```python
from build123d import *

# Parameters (mm, degrees)
SKETCH_1_W          = 42.04
SKETCH_1_H          = 27.22
EXTRUDE_1_DEPTH     = 0.52
SKETCH_3_W          = 42.04
SKETCH_3_H          = 23.01
EXTRUDE_2_DEPTH     = 0.71
SKETCH_5_W          = 35.05
SKETCH_5_H          = 15.32
CUT_EXTRUDE_1_DEPTH = 0.01
EXTRUDE_START       = -6.26
EXTRUDE_1_2_DEPTH   = 12.52


# Read off the part's stored shape, not the designer's step: 拉伸-薄壁1
with BuildPart() as part:
    # 草图1 → Extrude 1 (new body)
    with BuildSketch(Plane.XY):
        Rectangle(SKETCH_1_W, SKETCH_1_H)
    extrude(amount=EXTRUDE_1_DEPTH)

    # 草图3 → 凸台-拉伸2 (add)
    with BuildSketch(Plane.XY):
        with Locations((0, 2.105)):
            Rectangle(SKETCH_3_W, SKETCH_3_H)
    extrude(amount=-EXTRUDE_2_DEPTH)

    # 草图5 → 切除-拉伸1 (cut)
    with BuildSketch(Plane.XY):
        with Locations((0, 2.105)):
            Rectangle(SKETCH_5_W, SKETCH_5_H)
    extrude(amount=-CUT_EXTRUDE_1_DEPTH, mode=Mode.SUBTRACT)

    # Extrude 1 2 outline → Extrude 1 2 (add)
    with BuildSketch(Plane(origin=(0, 0, 0), x_dir=(0, 0, -1), z_dir=(1, 0, 0)).offset(EXTRUDE_START)):
        with BuildLine():
            Line((0, -13.61), (-0.1, -13.61))
            add(Edge.make_bspline(
                [(-0.1, -13.61), (-0.1, -13.811999948), (-0.062447397, -13.983759134), (0.087597414, -14.266880112), (0.200229868, -14.375905512), (0.61293299, -14.604541747), (0.98162629, -14.634564325), (2.275338874, -14.53538179), (3.401387146, -14.206264697), (4.808904257, -13.842712132), (5.090182683, -13.77233657), (5.643385338, -13.645546605), (5.91499808, -13.589621122), (6.715455086, -13.444072044), (7.229865116, -13.376385405), (8.718879461, -13.254443705), (9.639245367, -13.281281386), (12.212088444, -13.631316764), (13.676832265, -14.22370802), (16.256955878, -15.84390487), (17.371964057, -16.872230984), (20.403860489, -20.184886502), (22.003130479, -22.695949544), (24.648389829, -25.189380489), (25.574110216, -25.809694734), (27.660843497, -26.317217871), (28.817134045, -26.200070844), (30.142790661, -25.575336117)],
                knots=[0, 0, 0, 0, 0.015625, 0.015625, 0.03125, 0.03125, 0.0625, 0.0625, 0.125, 0.125, 0.140625, 0.140625, 0.15625, 0.15625, 0.1875, 0.1875, 0.25, 0.25, 0.375, 0.375, 0.5, 0.5, 0.75, 0.75, 0.875, 0.875, 1, 1, 1, 1], degree=3))
            Line((30.142790661, -25.575336117), (30.100160891, -25.484877824))
            add(Edge.make_bspline(
                [(0, -13.61), (0, -15.345647415), (20.557920243, -6.954998075), (21.119775691, -29.717013379), (30.100160891, -25.484877824)],
                knots=[0, 0, 0, 0, 0.142988606, 1, 1, 1, 1], degree=3))
        make_face()
    extrude(amount=EXTRUDE_1_2_DEPTH)


solid = part.part
```
CAD build for the part. Positions are in the model's coordinates, mm. A direction names the side the tool comes from. Give positions to 0.01 mm unless a question says otherwise; leave off trailing zeros. Loops run counter-clockwise (first coordinate to the right, second up) from the corner with the lowest first, then second, coordinate; pieces in that order, holes last. Notation, with made-up numbers: (41.25, 64) -> (53.25, 64) arc R16 ccw to (53.25, 83) -> close; hole circle Ø2 at (70, -22.75). An arc over 180 degrees is marked (long way). Use a Markdown table: item, result.
1. Wall check: L1, parallel to Z at x = 13, y = -11; L2, parallel to Z at x = 13, y = 11.5; L3, parallel to Y at x = 3.5, z = -23. Give the ranges that are in metal, low to high. Write a range as [from, to].
Check result:
| item | result |
|---|---|
| L1 | z = [0, 0.52] |
| L2 | z = [-0.71, 0.52] |
| L3 | y = [-23.58, -23.43] |
2. Flat gauge pins, fed straight in: pin 1 (17 mm diameter, centred on x = 4.5, y = 2, fed in from -Z); pin 2 (14.5 mm diameter, centred on y = -21.5, z = -18.5, fed in from +X); pin 3 (3 mm diameter, centred on x = -6, z = -19.5, fed in from +Y). Where does each tip first touch, or does it go through?
Check result:
| item | result |
|---|---|
| pin 1 | stops at z = -0.71 |
| pin 2 | stops at x = 6.26 |
| pin 3 | stops at y = -17.42 |
3. Slice it at B-B (x = 7.5). List the corners of the cut face in (y, z) (3 decimals).
Check result:
| item | result |
|---|---|
| outline | (-13.61, 0) -> (-9.4, 0) -> (-9.4, -0.71) -> (13.61, -0.71) -> (13.61, 0.52) -> (-13.61, 0.52) -> close; hole (-5.555, -0.01) -> (9.765, -0.01) -> (9.765, 0) -> (-5.555, 0) -> close |
4. Which spindle directions (+Z, -Z, +X, -X, +Y, -Y) get a long thin tool onto all of the face, cutting with end or side? Do faces 1 (the flat face through (0, 2, -0.71)), 2 (the flat face through (0, 13.61, 0)). Say none if no direction does.
Check result:
| item | result |
|---|---|
| face 1 | -Z, +X, -X, +Y |
| face 2 | +Z, -Z, +X, -X, +Y |
5. Slice it at A-A (y = -1). List the corners of the cut face in (x, z) (3 decimals), plus the area to 3 significant figures.
Check result:
| item | result |
|---|---|
| outline | (-21.02, -0.71) -> (21.02, -0.71) -> (21.02, 0.52) -> (-21.02, 0.52) -> close; hole (-17.525, -0.01) -> (17.525, -0.01) -> (17.525, 0) -> (-17.525, 0) -> close |
| area | 51.4 mm^2 |
